```python
from build123d import *

# Parameters (mm, degrees)
EXTRUDE_2_DEPTH     = 3
EXTRUDE_3_DEPTH     = 20
SKETCH_5_R          = 2.25
SKETCH_5_R_2        = 2.5
CUT_EXTRUDE_1_DEPTH = 98.430183655


with BuildPart() as part:
    # 草图2 → 凸台-拉伸2 (new body)
    with BuildSketch(Plane(origin=(0, 0, 0), x_dir=(1, 0, 0), z_dir=(0, 1, 0))):
        with BuildLine():
            Line((-58.569449541, 23.337085947), (32.740581269, -53.879999426))
            ThreePointArc((32.740581269, -53.879999426), (53.033008589, -53.033008589), (53.879999426, -32.740581269))
            Line((53.879999426, -32.740581269), (-23.337085947, 58.569449541))
            ThreePointArc((-23.337085947, 58.569449541), (-60.104076401, 60.104076401), (-58.569449541, 23.337085947))
        make_face()
    extrude(amount=EXTRUDE_2_DEPTH)

    # 草图4 → 凸台-拉伸3 (add)
    with BuildSketch(Plane(origin=(0, 3, 0), x_dir=(1, 0, 0), z_dir=(0, 1, 0))):
        with BuildLine():
            ThreePointArc((-23.337085947, 58.569449541), (-60.104076401, 60.104076401), (-58.569449541, 23.337085947))
            Line((-58.569449541, 23.337085947), (32.740581269, -53.879999426))
            ThreePointArc((32.740581269, -53.879999426), (53.033008589, -53.033008589), (53.879999426, -32.740581269))
            Line((53.879999426, -32.740581269), (-23.337085947, 58.569449541))
        make_face()
        with BuildLine():
            ThreePointArc((-56.632284421, 25.627804458), (-57.982756057, 57.982756057), (-25.627804458, 56.632284421))
            Line((-25.627804458, 56.632284421), (51.589280915, -34.67774639))
            ThreePointArc((51.589280915, -34.67774639), (50.911688245, -50.911688245), (34.67774639, -51.589280915))
            Line((34.67774639, -51.589280915), (-56.632284421, 25.627804458))
        make_face(mode=Mode.SUBTRACT)
    extrude(amount=EXTRUDE_3_DEPTH)

    # 草图5 → 切除-拉伸1 (cut, through all)
    with BuildSketch(Plane(origin=(0, 3, 0), x_dir=(1, 0, 0), z_dir=(0, 1, 0))):
        with Locations(Location((-42.426406871, 42.426406871, 0), (0, 0, 270))):
            Circle(SKETCH_5_R)
        with Locations(Location((42.426406871, -42.426406871, 0), (0, 0, 270))):
            Circle(SKETCH_5_R_2)
    extrude(amount=-CUT_EXTRUDE_1_DEPTH, mode=Mode.SUBTRACT)


solid = part.part
```
Work out the finished part from the listing and answer in its coordinate system (mm). A direction names the side the tool comes from. Give positions to 0.01 mm unless a question says otherwise; leave off trailing zeros. Write each loop counter-clockwise with the first axis right and the second up, starting at its lowest first coordinate (ties: lowest second). Pieces come first, ordered by that corner, then holes.
(1) The part is cut by section B-B on x = -10.5. Write down the section's boundary in (y, z), plus the area to 3 significant figures.
Final values:
outline: (0, -43.39) - (23, -43.39) - (23, -38.74) - (3, -38.74) - (3, 13.38) - (23, 13.38) - (23, 17.31) - (0, 17.31) - close
area: 354 mm2
(2) The part is cut by section A-A on y = 11. Write down the section's boundary in (x, z), plus the area to 3 significant figures.
Final values:
outline: (-58.57, -23.34) arc R25 ccw (long way) to (-23.34, -58.57) - (53.88, 32.74) arc R15 ccw to (32.74, 53.88) - close; hole (-56.63, -25.63) arc R22 ccw (long way) to (-25.63, -56.63) - (51.59, 34.68) arc R12 ccw to (34.68, 51.59) - close
area: 1,070 mm2
(3) Straight lines are drawn through the part: line 1 (Y direction, x = -6.5, z = -24.5); line 2 (X direction, y = 21.5, z = 39.5); line 3 (X direction, y = 11.5, z = 28.5). For each, find the intervals that lie inside material, in ascending order.
Final values:
line 1: y = 0 to 3
line 2: x = 15.74 to 20.38, 54.06 to 57.14
line 3: x = 2.73 to 7.37, 46.37 to 50.29
(4) Flat-ended cylindrical pins translate along their axes: pin 1 Ø10 at (y, z) = (16, -19.5) entering from +X; pin 2 Ø4 at (y, z) = (14.5, 28) entering from +X; pin 3 Ø6 at (y, z) = (14, 37.5) entering from +X. Find the tip coordinate at first contact, or state that the pin passes through.
Final values:
pin 1: stops at x = 13.93
pin 2: stops at x = 51.56
pin 3: stops at x = 57.3
(5) The part is cut by section C-C on z = 6.5. Write down the section's boundary in (x, y), plus the area to 3 significant figures.
Final values:
outline: (-23.29, 0) - (31.69, 0) - (31.69, 23) - (27.76, 23) - (27.76, 3) - (-18.64, 3) - (-18.64, 23) - (-23.29, 23) - close
area: 336 mm2
(6) The mould has two halves that part along X. Classify faces 3 (the flat face through (-13.554, 11.339, 14.731)), 4 (the flat face through (15.81, 11.34, -12.28)), 5 (the flat face through (-6, 3, -6)), 6 (the flat face through (-6, 0, -6)): pulls with the +X half, pulls with the -X half, needs draft (parallel to the pull), parting line crosses it, or undercut.
Final values:
face 3: pulls with the -X half
face 4: pulls with the +X half
face 5: undercut
face 6: needs draft
(7) Which of the six approach directions +Z, -Z, +X, -X, +Y, -Y give full straight-line access (tool end or side, diameter ignored) to faces 1 (the cylindrical face through (-59.7, 11.3, -60.5)), 2 (the cylindrical face through (51.09, 12.86, 50.73))?
Final values:
face 1: +Y, -Y
face 2: +Y
